Read the model definition and answer for the solid it produces. Units are mm, in the model's axes. A direction names the side the tool comes from. Give positions to 0.01 mm unless a question says otherwise; leave off trailing zeros. Write each loop counter-clockwise with the first axis right and the second up, starting at its lowest first coordinate (ties: lowest second). Pieces come first, ordered by that corner, then holes.
```python
from build123d import *

# Parameters (mm, degrees)
SKETCH1_R           = 2.15
SKETCH1_R_2         = 6.3
BOSS_EXTRUDE1_DEPTH = 4
FILLET1_R           = 2
CHAMFER1_SIZE       = 0.4


with BuildPart() as part:
    # Sketch1 → Boss-Extrude1 (new body)
    with BuildSketch(Plane.XY):
        Polygon((0, -50), (30, -50), (30, -30), (50, -30), (50, 0), (0, 0), align=None)
        with Locations((15, -40)):
            Circle(SKETCH1_R, mode=Mode.SUBTRACT)
        with Locations((40, -15)):
            Circle(SKETCH1_R, mode=Mode.SUBTRACT)
        with Locations((22.928932188, -22.928932188)):
            Circle(SKETCH1_R_2, mode=Mode.SUBTRACT)
    extrude(amount=BOSS_EXTRUDE1_DEPTH)

    # Fillet1
    fillet1_edges = [part.edges().sort_by_distance(p)[0] for p in [
        (0, 0, 2),
        (50, 0, 2),
        (50, -30, 2),
        (30, -50, 2),
        (0, -50, 2),
    ]]
    fillet(fillet1_edges, radius=FILLET1_R)

    # Chamfer1
    chamfer1_edges = [part.edges().sort_by_distance(p)[0] for p in [
        (39, -30, 4),
        (12.85, -40, 0),
        (12.85, -40, 4),
        (37.85, -15, 0),
        (37.85, -15, 4),
        (16.628932188, -22.928932188, 0),
        (16.628932188, -22.928932188, 4),
        (0, -25, 0),
        (0, -25, 4),
        (25, 0, 0),
        (50, -15, 0),
        (30, -39, 0),
        (15, -50, 0),
        (29.414213562, -49.414213562, 0),
        (0.585786438, -49.414213562, 0),
        (49.414213562, -29.414213562, 0),
        (49.414213562, -0.585786438, 0),
        (0.585786438, -0.585786438, 0),
        (25, 0, 4),
        (15, -50, 4),
        (30, -39, 4),
        (50, -15, 4),
        (29.414213562, -49.414213562, 4),
        (0.585786438, -49.414213562, 4),
        (49.414213562, -29.414213562, 4),
        (49.414213562, -0.585786438, 4),
        (0.585786438, -0.585786438, 4),
        (39, -30, 0),
    ]]
    chamfer(chamfer1_edges, length=CHAMFER1_SIZE)


solid = part.part
```
Item 1: Find the intervals of material crossed by line 1 along Y through (x, z) = (40, 2.5); line 2 along Y through (x, z) = (15, 2); line 3 along X through (y, z) = (-37, 1.55), in increasing order.
Result set:
line 1: y = -30 to -17.15, -12.85 to 0
line 2: y = -50 to -42.15, -37.85 to 0
line 3: x = 0 to 30
Item 2: Determine the mould class of faces 1 (the cylindrical face through (29.4, -49.43, 2.02)), 2 (the flat face through (30, -39, 2)), 3 (the cylindrical face through (28.94, -21.04, 1.98)), 4 (the cylindrical face through (49.4, -0.57, 2.02)) for opening direction Y: pulls with the +Y half, pulls with the -Y half, needs draft (parallel to the pull), parting line crosses it, or undercut.
Result set:
face 1: pulls with the -Y half
face 2: needs draft
face 3: undercut
face 4: pulls with the +Y half
Item 3: Which of the six approach directions +Z, -Z, +X, -X, +Y, -Y give full straight-line access (tool end or side, diameter ignored) to faces 5 (the flat face through (15, -50, 2)), 6 (the flat face through (39, -30, 2))?
Result set:
face 5: +Z, -Z, +X, -X, -Y
face 6: +Z, -Z, +X, -Y
Item 4: Section C-C (z = 1.6) is taken. Write down the section's boundary in (x, y).
Result set:
outline: (0, -48) arc R2 ccw to (2, -50) - (28, -50) arc R2 ccw to (30, -48) - (30, -30) - (48, -30) arc R2 ccw to (50, -28) - (50, -2) arc R2 ccw to (48, 0) - (2, 0) arc R2 ccw to (0, -2) - close; hole circle Ø4.3 at (15, -40); hole circle Ø12.6 at (22.93, -22.93); hole circle Ø4.3 at (40, -15)
Item 5: This flat-tipped pin is pushed along its axis until it touches: pin 1 Ø1.6 at (y, z) = (-35, 2.5) entering from +X. Where does it stop, or does it pass through?
Result set:
pin 1: stops at x = 30
Item 6: Section A-A (x = 40) is taken. Write down the section's boundary in (y, z).
Result set:
outline: (-30, 0.4) - (-29.6, 0) - (-17.55, 0) - (-17.15, 0.4) - (-17.15, 3.6) - (-17.55, 4) - (-29.6, 4) - (-30, 3.6) - close; (-12.85, 0.4) - (-12.45, 0) - (-0.4, 0) - (0, 0.4) - (0, 3.6) - (-0.4, 4) - (-12.45, 4) - (-12.85, 3.6) - close
Item 7: Section D-D (y = -36) is taken. Write down the section's boundary in (x, z), and give its area (3 significant figures).
Result set:
outline: (0, 0.4) - (0.4, 0) - (29.6, 0) - (30, 0.4) - (30, 3.6) - (29.6, 4) - (0.4, 4) - (0, 3.6) - close
area: 120 mm2
Item 8: Section B-B (y = -15) is taken. Write down the section's boundary in (x, z).
Result set:
outline: (0, 0.4) - (0.4, 0) - (37.45, 0) - (37.85, 0.4) - (37.85, 3.6) - (37.45, 4) - (0.4, 4) - (0, 3.6) - close; (42.15, 0.4) - (42.55, 0) - (49.6, 0) - (50, 0.4) - (50, 3.6) - (49.6, 4) - (42.55, 4) - (42.15, 3.6) - close
